Design review of the part built by this model. Coordinates are the model's own, in mm. Round coordinates to 2 decimals unless told otherwise and drop trailing zeros. Loops run counter-clockwise (first coordinate to the right, second up) from the corner with the lowest first, then second, coordinate; pieces in that order, holes last. Notation, with made-up numbers: M -29,71.25 L 3,71.25 A19 ccw 3,97.25 Z; hole C 54.25,19 d10. An arc over 180 degrees is marked long. Use a Markdown table: item, result.
from build123d import *

# Parameters (mm, degrees)
F1_DEPTH = 0.9
F2_R     = 5
F4_DEPTH = 0.9
F5_R     = 3


with BuildPart() as f1:
    # F0 (on Top) → F1 (new body)
    with BuildSketch(Plane.XY):
        Polygon((43.3012701892, -25), (43.3012701892, 25), (0, 50), (-43.3012701892, 25), (-43.3012701892, -25), (0, -50), align=None)
        Polygon((0, 44.2264973081), (38.3012701892, 22.1132486541), (38.3012701892, -22.1132486541), (0, -44.2264973081), (-38.3012701892, -22.1132486541), (-38.3012701892, 22.1132486541), align=None, mode=Mode.SUBTRACT)
    extrude(amount=F1_DEPTH)

    # F2
    f2_edges = [f1.edges().sort_by_distance(p)[0] for p in [
        (0, 50, 0.45),
        (43.30127, 25, 0.45),
        (-43.30127, 25, 0.45),
        (-43.30127, -25, 0.45),
        (0, -50, 0.45),
        (43.30127, -25, 0.45),
    ]]
    fillet(f2_edges, radius=F2_R)

    # F3 (on Top) → F4 (join, through all)
    with BuildSketch(Plane.XY):
        Polygon((0, 5), (-19.4855715851, 38.75), (-23.8156986041, 36.25), (-4.3301270189, 2.5), (-1.443375673, 2.5), align=None)
        Polygon((19.4855715851, 38.75), (0, 5), (1.443375673, 2.5), (4.3301270189, 2.5), (23.8156986041, 36.25), align=None)
        Polygon((1.443375673, 2.5), (0, 5), (-1.443375673, 2.5), align=None)
        Polygon((-1.443375673, 2.5), (-4.3301270189, 2.5), (-2.8867513459, 0), align=None)
        Polygon((-2.8867513459, 0), (-4.3301270189, 2.5), (-43.3012701892, 2.5), (-43.3012701892, -2.5), (-4.3301270189, -2.5), align=None)
        Polygon((4.3301270189, 2.5), (1.443375673, 2.5), (2.8867513459, 0), align=None)
        Polygon((-1.443375673, -2.5), (-2.8867513459, 0), (-4.3301270189, -2.5), align=None)
        Polygon((4.3301270189, 2.5), (2.8867513459, 0), (4.3301270189, -2.5), (43.3012701892, -2.5), (43.3012701892, 2.5), align=None)
        Polygon((4.3301270189, -2.5), (2.8867513459, 0), (1.443375673, -2.5), align=None)
        Polygon((1.443375673, -2.5), (-1.443375673, -2.5), (0, -5), align=None)
        Polygon((0, -5), (-1.443375673, -2.5), (-4.3301270189, -2.5), (-23.8156986041, -36.25), (-19.4855715851, -38.75), align=None)
        Polygon((23.8156986041, -36.25), (4.3301270189, -2.5), (1.443375673, -2.5), (0, -5), (19.4855715851, -38.75), align=None)
    extrude(amount=F4_DEPTH)

    # F5
    f5_edges = [f1.edges().sort_by_distance(p)[0] for p in [
        (-4.330127, -2.5, 0.45),
        (-4.330127, 2.5, 0.45),
        (0, 5, 0.45),
        (0, -5, 0.45),
        (4.330127, -2.5, 0.45),
        (4.330127, 2.5, 0.45),
    ]]
    fillet(f5_edges, radius=F5_R)


solid = f1.part
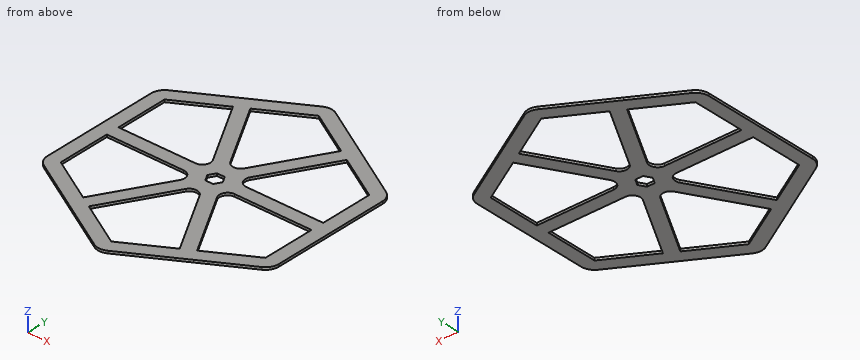
1. Take a section at B-B on y = -37.5. Give the boundary of the cut face in (x, z).
Check values:
| item | result |
|---|---|
| outline | M -21.65,0 L -11.65,0 L -11.65,0.9 L -21.65,0.9 Z; M 11.65,0 L 21.65,0 L 21.65,0.9 L 11.65,0.9 Z |
2. Wall thickness on line 1 along X through (y, z) = (-5.5, 0.1); line 2 along X through (y, z) = (-7.5, 0.65); line 3 along Y through (x, z) = (-12.5, 0.4): over which ranges is each line inside the solid? List them lowest first. Write a range as from..to.
Check values:
| item | result |
|---|---|
| line 1 | x = -43.3..-38.3, -6.53..6.53, 38.3..43.3 |
| line 2 | x = -43.3..-38.3, -7.22..7.22, 38.3..43.3 |
| line 3 | y = -42.78..-37.01, -26.65..-16.65, -2.5..2.5, 16.65..26.65, 37.01..42.78 |
3. Take a section at C-C on x = 8. Give the boundary of the cut face in (y, z), and give its area (3 significant figures).
Check values:
| item | result |
|---|---|
| outline | M -45.38,0 L -39.61,0 L -39.61,0.9 L -45.38,0.9 Z; M -18.86,0 L -8.86,0 L -8.86,0.9 L -18.86,0.9 Z; M -2.92,0 L 2.92,0 L 2.92,0.9 L -2.92,0.9 Z; M 8.86,0 L 18.86,0 L 18.86,0.9 L 8.86,0.9 Z; M 39.61,0 L 45.38,0 L 45.38,0.9 L 39.61,0.9 Z |
| area | 33.6 mm² |
4. Take a section at D-D on y = 29. Give the boundary of the cut face in (x, z).
Check values:
| item | result |
|---|---|
| outline | M -36.37,0 L -26.37,0 L -26.37,0.9 L -36.37,0.9 Z; M -19.63,0 L -13.86,0 L -13.86,0.9 L -19.63,0.9 Z; M 13.86,0 L 19.63,0 L 19.63,0.9 L 13.86,0.9 Z; M 26.37,0 L 36.37,0 L 36.37,0.9 L 26.37,0.9 Z |
5. Take a section at A-A on x = -31.5. Give the boundary of the cut face in (y, z), and give its area (3 significant figures).
Check values:
| item | result |
|---|---|
| outline | M -31.81,0 L -26.04,0 L -26.04,0.9 L -31.81,0.9 Z; M -2.5,0 L 2.5,0 L 2.5,0.9 L -2.5,0.9 Z; M 26.04,0 L 31.81,0 L 31.81,0.9 L 26.04,0.9 Z |
| area | 14.9 mm² |
